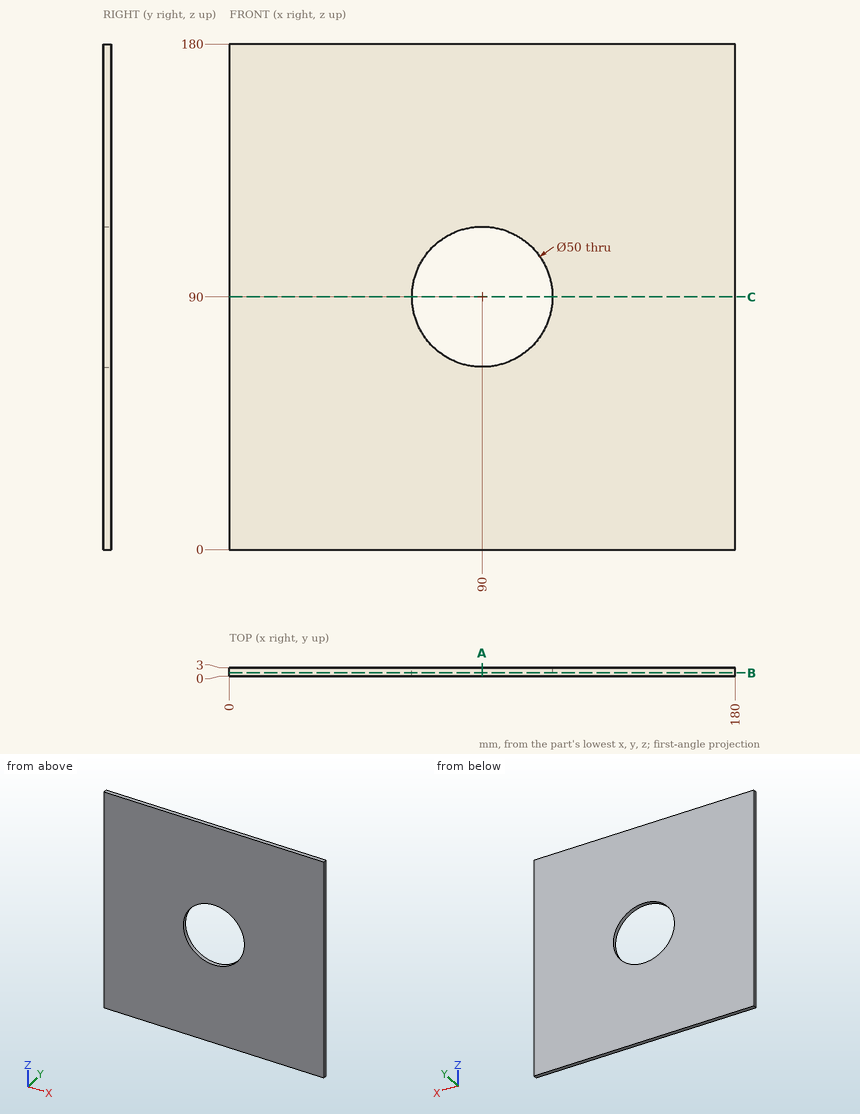
Study the drawing (mm; zero at the part's minimum x, y, z) and answer. Give positions to 0.01 mm unless a question says otherwise; leave off trailing zeros. Order: outer loops, then holes, each group sorted by start corner. A loop starts at its lowest first (then second) coordinate and runs counter-clockwise, first axis right, second up. Notation, with made-up numbers: (-35, 57.5) - (11, 57.5) arc R17 cw to (11, 84.5) - close; hole circle Ø8 at (-10.5, -27.5). An arc over 180 degrees is marked (long way). Answer in a Markdown table with one row per item. Add a question column.
Q1. Find the intervals of material crossed by line 1 along Z through (x, y) = (90, 1.2); line 2 along Z through (x, y) = (80, 1.65), in increasing order. Write a range as [from, to].
Q2. The part is cut by section C-C (z = 90). Determine the outline of the cut face in (x, y), then the cut area to 3 significant figures.
Q3. The part is cut by section A-A (x = 90). Determine the outline of the cut face in (y, z).
Q4. The part is cut by section B-B (y = 1.1). Determine the outline of the cut face in (x, z), then the cut area to 3 significant figures.
Determined:
| question | item | result |
|---|---|---|
| 1 | line 1 | z = [0, 65], [115, 180] |
| 1 | line 2 | z = [0, 67.09], [112.91, 180] |
| 2 | outline | (0, 0) - (65, 0) - (65, 3) - (0, 3) - close; (115, 0) - (180, 0) - (180, 3) - (115, 3) - close |
| 2 | area | 390 mm² |
| 3 | outline | (0, 0) - (3, 0) - (3, 65) - (0, 65) - close; (0, 115) - (3, 115) - (3, 180) - (0, 180) - close |
| 4 | outline | (0, 0) - (180, 0) - (180, 180) - (0, 180) - close; hole circle Ø50 at (90, 90) |
| 4 | area | 30,400 mm² |
